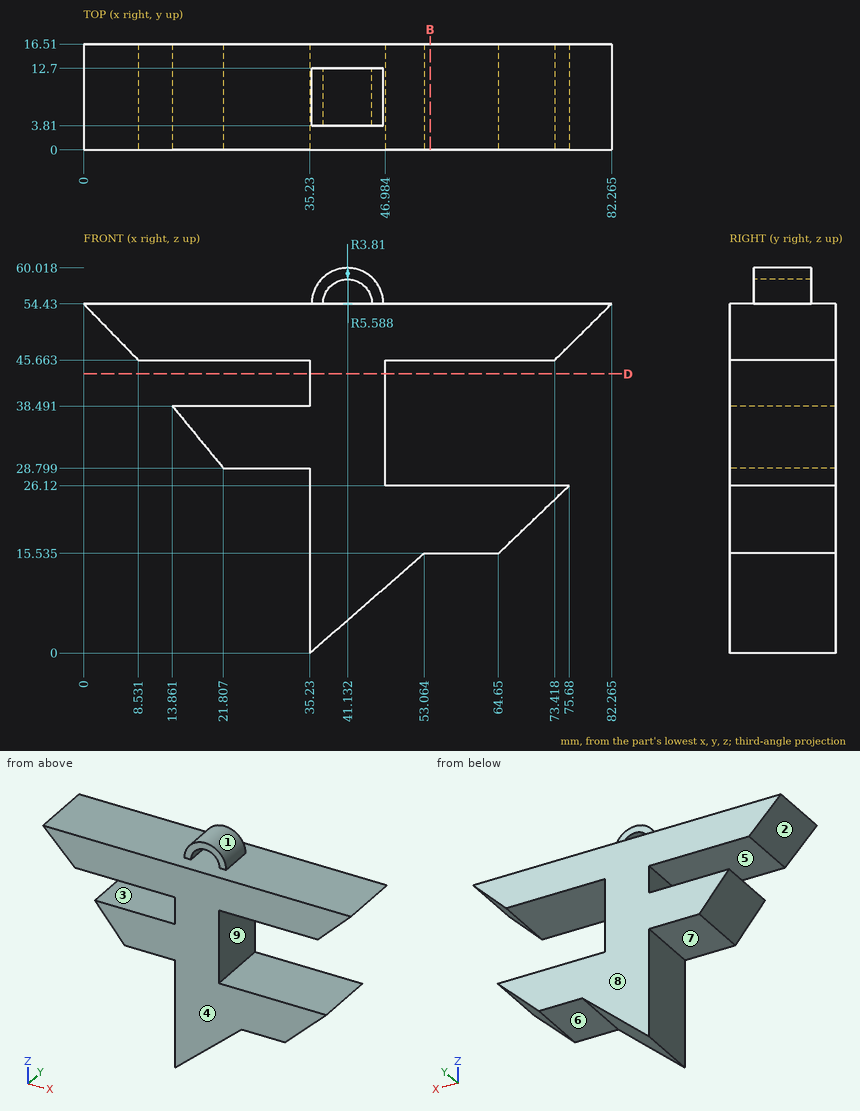
Source: three-view drawing plus pictorial views. Frame: mm from the lowest corner of the part. A direction names the side the tool comes from. Give positions to 0.01 mm unless a question says otherwise; leave off trailing zeros. Write each loop counter-clockwise with the first axis right and the second up, starting at its lowest first coordinate (ties: lowest second). Pieces come first, ordered by that corner, then holes.
(1) First-contact query: P1, Ø3, axis at x = 42.5, z = 57, coming from the -Y side; P2, Ø4, axis at y = 11, z = 46.5, coming from the -X side; P3, Ø4, axis at y = 12, z = 40, coming from the -X side. Flat tips, straight axial feed; report the tip coordinate or a pass-through.
(2) Cut plane B-B, the plane x = 54. Return loops of the section in (y, z) (1 decimal).
(3) Cut plane D-D, the plane z = 43.5. Return loops of the section in (x, y) (1 decimal).
(4) Mould query, pull axis Z, two halves, no side actions, for the marked faces 1, 2, 3 and 4. Classes: released by +Z, released by -Z, zero draft, split by the parting line, or undercut.
(5) Access query for the marked faces 5, 6, 7, 8 and 9. Directions: +Z, -Z, +X, -X, +Y, -Y. A direction counts if a zero-diameter tool reaches every point of the face in a straight line with its end or side. Return the directions, or none.
(6) Ray query, line 1 (Z direction, x = 26, y = 12.5); line 2 (Z direction, x = 61, y = 3) (1 decimal); line 3 (X direction, y = 2, z = 28) (1 decimal). Return the intervals inside material, ascending.
Values follow:
1. P1: stops at y = 3.81
1. P2: stops at x = 5.77
1. P3: stops at x = 13.86
2. outline: (0, 15.5) - (16.5, 15.5) - (16.5, 26.1) - (0, 26.1) - close; (0, 45.7) - (16.5, 45.7) - (16.5, 54.4) - (0, 54.4) - close
3. outline: (35.2, 0) - (47, 0) - (47, 16.5) - (35.2, 16.5) - close
4. face 1: released by +Z
4. face 2: released by -Z
4. face 3: undercut
4. face 4: zero draft
5. face 5: -X, +Y, -Y
5. face 6: -Z, +X, +Y, -Y
5. face 7: -Z, -X, +Y, -Y
5. face 8: +Z, -Z, +X, -X, +Y
5. face 9: +X, +Y, -Y
6. line 1: z = 28.8 to 38.49, 45.66 to 54.43
6. line 2: z = 15.5 to 26.1, 45.7 to 54.4
6. line 3: x = 35.2 to 47
